Autodesk Inventor part; units mm, degrees
ref_plane "YZ Plane" through (0, 0, 0) normal (1, 0, 0) x (0, 1, 0)
ref_plane "XZ Plane" through (0, 0, 0) normal (0, 1, 0) x (-1, 0, 0)
ref_plane "XY Plane" through (0, 0, 0) normal (0, 0, 1) x (1, 0, 0)
sketch "Sketch1" plane through (0, 0, 0) normal (0, 1, 0) x (-1, 0, 0)
  line L0 (0, 0) -> (-15.24, 0)
  line L1 (-15.24, 0) -> (-15.24, -15.24)
  line L2 (-15.24, -15.24) -> (0, -15.24)
  line L3 (0, -15.24) -> (0, 0)
  dimension "d0" = 15.24
  dimension "d1" = 15.24
extrude "Extrusion1" add sketch "Sketch1" along normal blind 1.27
sketch "Sketch2" plane through (0, 1.27, 0) normal (0, 1, 0) x (1, 0, 0)
  line L0 (0, 15.24) -> (0, 0)
  line L1 (0, 15.24) -> (1.524, 15.24)
  line L2 (1.524, 15.24) -> (1.524, 7.366)
  line L3 (1.524, 7.366) -> (0, 7.366)
  line L4 (0, 7.366) -> (0, 15.24)
  line L5 (15.24, 0) -> (15.24, 15.24)
  line L6 (15.24, 15.24) -> (13.716, 15.24)
  line L7 (13.716, 15.24) -> (13.716, 7.366)
  line L8 (13.716, 7.366) -> (15.24, 7.366)
  line L9 (15.24, 7.366) -> (15.24, 15.24)
  dimension "d4" = 1.524
  dimension "d5" = 7.874
  dimension "d6" = 1.524
  dimension "d7" = 7.874
fillet "Fillet1" radius 1.016 4 edges at (7.62, 1.27, 0) (7.62, 1.27, -15.24) (15.24, 1.27, -7.62) (0, 1.27, -7.62)
hole "Hole2" at (1.524, 1.27, -7.366) at (13.716, 1.27, -7.366) direction (0, -1, 0) diameter 3.048 end through all
properties part number "Cap"
Check sheet for the modelled part. Datum: model origin and axes. Units: mm. Give positions to 0.01 mm unless a question says otherwise; leave off trailing zeros. Loops run counter-clockwise (first coordinate to the right, second up) from the corner with the lowest first, then second, coordinate; pieces in that order, holes last. Notation, with made-up numbers: M 43.5,75.25 L 71.5,75.25 A16 ccw 71.5,88.25 Z; hole C -23.5,85 d6. An arc over 180 degrees is marked long. Return JSON: item names as keys, results as strings. Group by question number.
1. Cross-section at C-C on y = 1. Record the boundary of the cut face in (x, z).
2. Go/stop test with a flat-tipped pin: pin 1 (1 mm diameter, centred on x = 7.5, z = -6, fed in from -Y). Record where the tip stops, or that it passes through.
3. Cross-section at A-A on x = 12.75. Record the boundary of the cut face in (y, z), plus the area to 3 significant figures.
4. Thickness scan on L1, parallel to X at y = 0.4, z = -6.5; L2, parallel to Z at x = 1.75, y = 0.55; L3, parallel to Z at x = 2, y = 1.1. Record the ranges inside material, lowest first.
5. Cross-section at B-B on z = -3. Record the boundary of the cut face in (x, y), plus the area to 3 significant figures.
6. Cross-section at D-D on z = -7. Record the boundary of the cut face in (x, y), plus the area to 3 significant figures.
Return value:
{
 "1": {"outline": "M 0.33,-14.91 L 14.91,-14.91 L 14.91,-8.31 A1.52 cw long 14.91,-6.42 L 14.91,-0.33 L 0.33,-0.33 L 0.33,-6.42 A1.52 cw long 0.33,-8.31 Z"},
 "2": {"pin 1": "y = 0"},
 "3": {"outline": "M 0,-15.24 L 0.25,-15.24 A1.02 ccw 1.27,-14.22 L 1.27,-8.54 L 0,-8.54 Z; M 0,-6.19 L 1.27,-6.19 L 1.27,-1.02 A1.02 ccw 0.25,0 L 0,0 Z", "area": "15.9 mm^2"},
 "4": {"L1": "0.01 to 0.27, 2.78 to 12.46, 14.97 to 15.23", "L2": "-15.2 to -8.87, -5.86 to -0.04", "L3": "-14.79 to -8.81, -5.92 to -0.45"},
 "5": {"outline": "M 0,0 L 15.24,0 L 15.24,0.25 A1.02 ccw 14.22,1.27 L 1.02,1.27 A1.02 ccw 0,0.25 Z", "area": "18.9 mm^2"},
 "6": {"outline": "M 0,0 L 0.04,0 L 0.04,0.55 A1.02 ccw 0,0.25 Z; M 3,0 L 12.24,0 L 12.24,1.27 L 3,1.27 Z; M 15.2,0 L 15.24,0 L 15.24,0.25 A1.02 ccw 15.2,0.55 Z", "area": "11.8 mm^2"}
}
